```python
from build123d import *

# Parameters (mm, degrees)
SKETCH1_R           = 12.5
BOSS_EXTRUDE2_DEPTH = 2
SKETCH2_R           = 12.5
SKETCH2_R_2         = 11.5
BOSS_EXTRUDE3_DEPTH = 10
REVOLVE1_ANGLE      = 30
CHAMFER1_SIZE       = 0.5
CHAMFER2_SIZE       = 0.75


with BuildPart() as part:
    # Sketch1 → Boss-Extrude2 (new body)
    with BuildSketch(Plane(origin=(0, 0, 0), x_dir=(1, 0, 0), z_dir=(0, 1, 0))):
        with Locations(Location((0, 0, 0), (0, 0, 270))):
            Circle(SKETCH1_R)
    extrude(amount=BOSS_EXTRUDE2_DEPTH)

    # Sketch2 → Boss-Extrude3 (add)
    with BuildSketch(Plane(origin=(0, 2, 0), x_dir=(1, 0, 0), z_dir=(0, 1, 0))):
        with Locations(Location((0, 0, 0), (0, 0, 270))):
            Circle(SKETCH2_R)
        with Locations(Location((0, 0, 0), (0, 0, 270))):
            Circle(SKETCH2_R_2, mode=Mode.SUBTRACT)
    extrude(amount=BOSS_EXTRUDE3_DEPTH)

    # Sketch3 → Revolve1 (revolve)
    with BuildSketch(Plane.XY):
        with BuildLine():
            Line((-11.5, 9.5), (-11.5, 7.5))
            ThreePointArc((-11.5, 7.5), (-10.5, 8.5), (-11.5, 9.5))
        make_face()
        with BuildLine():
            Line((11.5, 9.5), (11.5, 7.5))
            ThreePointArc((11.5, 7.5), (10.5, 8.5), (11.5, 9.5))
        make_face()
    revolve(axis=Axis((0, 19.49850662, 0), (0, -1, 0)), revolution_arc=REVOLVE1_ANGLE)

    # Chamfer1
    chamfer1_edges = [part.edges().sort_by_distance(p)[0] for p in [
        (0, 0, -12.5),
    ]]
    chamfer(chamfer1_edges, length=CHAMFER1_SIZE)

    # Chamfer2
    chamfer2_edges = [part.edges().sort_by_distance(p)[0] for p in [
        (0, 2, -11.5),
    ]]
    chamfer(chamfer2_edges, length=CHAMFER2_SIZE)


solid = part.part
```
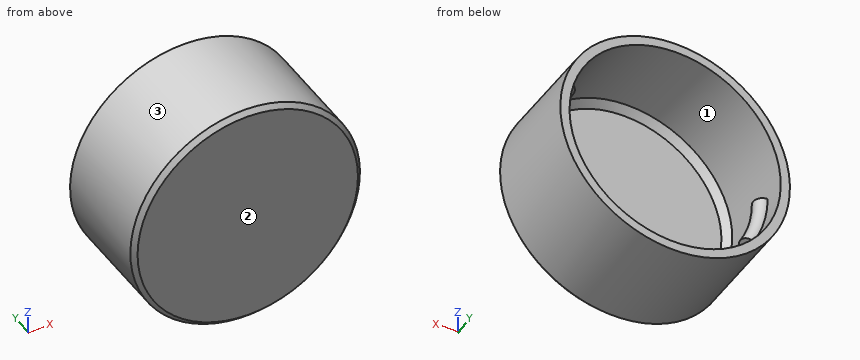
Verification items for the finished model (mm, model axes). Face numbers are marked on the shaded views. Give positions to 0.01 mm unless a question says otherwise; leave off trailing zeros. Loops run counter-clockwise (first coordinate to the right, second up) from the corner with the lowest first, then second, coordinate; pieces in that order, holes last.
1. Thickness scan on line 1 (X direction, y = 10.25, z = 0); line 2 (Y direction, x = 5.75, z = 4.5); line 3 (X direction, y = 3.25, z = 9.5). Record the ranges inside material, lowest first.
2. Go/stop test with flat-tipped pins: pin 1 Ø3 at (x, z) = (-9, -8) entering from -Y; pin 2 Ø1.5 at (x, y) = (-7.5, 1.5) entering from +Z; pin 3 Ø6 at (y, z) = (7.5, -4) entering from -X; pin 4 Ø1.1 at (x, y) = (-11, 9) entering from +Z. Record where each tip stops, or that it passes through.
3. Section check A-A, the plane x = 0. Enter the section's corners in (y, z).
4. Section check B-B, the plane y = 6.75. Enter the section's corners in (x, z), then the cut area to 3 significant figures.
5. Mould release check, pull along Z, two halves, no side actions. Record for the marked faces 1, 2 and 3: released by +Z, released by -Z, zero draft, split by the parting line, or undercut.
Geometry says:
1. line 1: x = -12.5 to -11.5, 11.5 to 12.5
1. line 2: y = 0 to 2
1. line 3: x = -8.12 to -6.48, 6.48 to 8.12
2. pin 1: stops at y = 0
2. pin 2: stops at z = 10.52
2. pin 3: stops at x = -12.46
2. pin 4: stops at z = 6.86
3. outline: (0, -12) - (0.5, -12.5) - (12, -12.5) - (12, -11.5) - (2.75, -11.5) - (2, -10.75) - (2, 10.75) - (2.75, 11.5) - (12, 11.5) - (12, 12.5) - (0.5, 12.5) - (0, 12) - close
4. outline: circle Ø25 at (0, 0); hole circle Ø23 at (0, 0)
4. area: 75.4 mm2
5. face 1: undercut
5. face 2: zero draft
5. face 3: split by the parting line
